Build history of the part. All positions in model axes, mm. Face numbers are marked on the shaded views. Round coordinates to 2 decimals unless told otherwise and drop trailing zeros. Order: outer loops, then holes, each group sorted by start corner. A loop starts at its lowest first (then second) coordinate and runs counter-clockwise, first axis right, second up. Notation, with made-up numbers: (16.25, 43) -> (25.25, 43) arc R22 cw to (25.25, 80) -> close; hole circle Ø2 at (75, 54). An arc over 180 degrees is marked (long way). Answer as a JSON object with one key per item and string values.
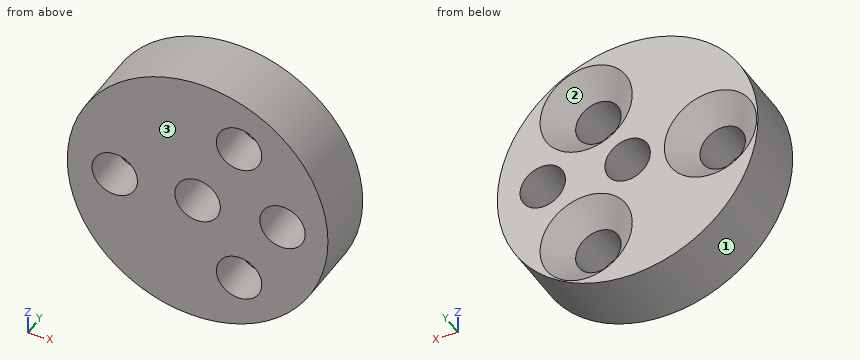
Autodesk Inventor part; units mm, degrees
ref_plane "YZ Plane" through (0, 0, 0) normal (1, 0, 0) x (0, 1, 0)
ref_plane "XZ Plane" through (0, 0, 0) normal (0, 1, 0) x (-1, 0, 0)
ref_plane "XY Plane" through (0, 0, 0) normal (0, 0, 1) x (1, 0, 0)
sketch "Szkic1" plane through (0, 0, 0) normal (0, 1, 0) x (-1, 0, 0)
  circle A0 centre (0, 0) radius 9.75
  dimension "d0" = 19.5
extrude "Wyciągnięcie proste1" add sketch "Szkic1" along normal blind 5
sketch "Szkic2" plane through (0, 5, 0) normal (0, 1, 0) x (1, 0, 0)
  line L0 (0, 0) -> (-6.2, 0) construction
  line L1 (0, 0) -> (3.1, 5.3694) construction
  line L2 (0, 0) -> (3.1, -5.3694) construction
  dimension "d3" = 6.2
  dimension "d4" = 120
  dimension "d5" = 120
hole "Otwór1" at (-6.2, 5, 0) at (3.1, 5, -5.3694) at (3.1, 5, 5.3694) direction (0, -1, 0) diameter 3.4 end through all countersink diameter 6.9 countersink angle 89.954
sketch "Szkic3" plane through (0, 5, 0) normal (0, 1, 0) x (1, 0, 0)
  line L0 (0, 0) -> (6.35, 0)
  dimension "d13" = 6.35
hole "Otwór2" at (0, 5, 0) at (6.35, 5, 0) direction (0, -1, 0) diameter 3.4 end through all
properties part number "PrzejsciowkaDoFormy"
1) Cut at A-A, the plane z = 0. Give the cut face in (x, y), plus the area to 3 significant figures.
Checked values:
{"outline": "(-9.75, 0) -> (-7.9, 0) -> (-7.9, 3.25) -> (-9.65, 5) -> (-9.75, 5) -> close; (-4.5, 0) -> (-1.7, 0) -> (-1.7, 5) -> (-2.75, 5) -> (-4.5, 3.25) -> close; (1.7, 0) -> (4.65, 0) -> (4.65, 5) -> (1.7, 5) -> close; (8.05, 0) -> (9.75, 0) -> (9.75, 5) -> (8.05, 5) -> close", "area": "43.4 mm²"}
2) Flat gauge pins, fed straight in: pin 1 Ø4 at (x, z) = (-6.2, 0) entering from +Y; pin 2 Ø2 at (x, z) = (3.1, 5.37) entering from -Y. Where does each tip first touch, or does it go through?
Checked values:
{"pin 1": "stops at y = 3.55", "pin 2": "passes through"}
3) Cut at D-D, the plane x = 3.1. Give the cut face in (y, z).
Checked values:
{"outline": "(0, -9.24) -> (5, -9.24) -> (5, -8.82) -> (3.25, -7.07) -> (0, -7.07) -> close; (0, -3.67) -> (3.25, -3.67) -> (5, -1.92) -> (5, 1.92) -> (3.25, 3.67) -> (0, 3.67) -> close; (0, 7.07) -> (3.25, 7.07) -> (5, 8.82) -> (5, 9.24) -> (0, 9.24) -> close"}
4) Cut at C-C, the plane x = -6.2. Give the cut face in (y, z), plus the area to 3 significant figures.
Checked values:
{"outline": "(0, -7.52) -> (5, -7.52) -> (5, -3.45) -> (3.25, -1.7) -> (0, -1.7) -> close; (0, 1.7) -> (3.25, 1.7) -> (5, 3.45) -> (5, 7.52) -> (0, 7.52) -> close", "area": "55.2 mm²"}
5) Pull direction Z, two halves, no side cores. Call the marked faces 1, 2 and 3: pulls with the +Z half, pulls with the -Z half, needs draft (parallel to the pull), parting line crosses it, or undercut.
Checked values:
{"face 1": "parting line crosses it", "face 2": "undercut", "face 3": "needs draft"}
6) Probe L1, parallel to X at y = 2.1, z = 1.5; L2, parallel to Z at x = 1.75, y = 2.9; L3, parallel to X at y = 3.9, z = -1.5. List the from-to ranges inside material, lowest first. Write a range as from..to.
Checked values:
{"L1": "x = -9.63..-7, -5.4..-0.8, 0.8..5.55, 7.15..9.63", "L2": "z = -9.59..-6.4, -4.34..4.34, 6.4..9.59", "L3": "x = -9.63..-8.01, -4.39..-0.8, 0.8..5.55, 7.15..9.63"}
7) Cut at B-B, the plane y = 1.3. Give the cut face in (x, z), plus the area to 3 significant figures.
Checked values:
{"outline": "circle Ø19.5 at (0, 0); hole circle Ø3.4 at (-6.2, 0); hole circle Ø3.4 at (0, 0); hole circle Ø3.4 at (3.1, -5.37); hole circle Ø3.4 at (3.1, 5.37); hole circle Ø3.4 at (6.35, 0)", "area": "253 mm²"}
